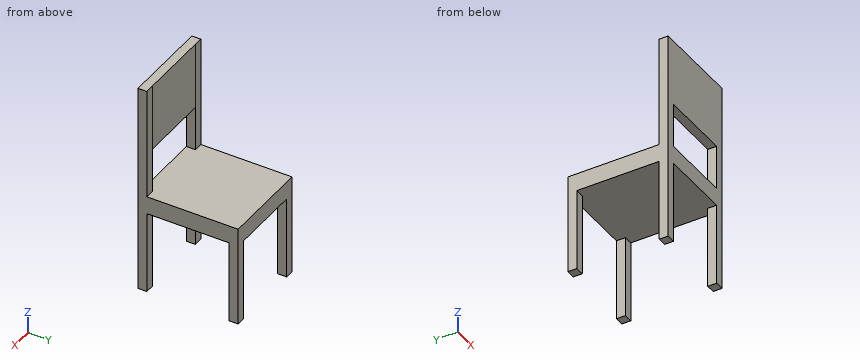
```python
from build123d import *

# Parameters (mm, degrees)
F0_W     = 400
F0_H     = 450
F1_DEPTH = 80
F2_W     = 40
F2_H     = 40
F3_DEPTH = 500
F4_DEPTH = 450
F5_W     = 360
F5_H     = 39.547034
F6_DEPTH = 300


with BuildPart() as f1:
    # F0 (on Top) → F1 (new body)
    with BuildSketch(Plane.XY):
        with Locations((200, 225)):
            Rectangle(F0_W, F0_H)
    extrude(amount=-F1_DEPTH)

    # F2 (on face) → F3 (join)
    with BuildSketch(Plane.XY):
        with Locations((20, 20)):
            Rectangle(F2_W, F2_H)
        with Locations((380, 20)):
            Rectangle(F2_W, F2_H)
    extrude(amount=F3_DEPTH)

    # F2 (on face) → F4 (join)
    with BuildSketch(Plane.XY):
        with Locations((20, 20)):
            Rectangle(F2_W, F2_H)
        with Locations((380, 20)):
            Rectangle(F2_W, F2_H)
        with Locations((380, 430)):
            Rectangle(F2_W, F2_H)
        with Locations((20, 430)):
            Rectangle(F2_W, F2_H)
    extrude(amount=-F4_DEPTH)

    # F5 (on face) → F6 (join)
    with BuildSketch(Plane.XY.offset(500)):
        with Locations((220, 19.773517)):
            Rectangle(F5_W, F5_H)
    extrude(amount=-F6_DEPTH)


solid = f1.part
```
Work out the finished part from the listing and answer in its coordinate system (mm). Coordinates: 2 decimals unless noted, no trailing zeros. Order: outer loops, then holes, each group sorted by start corner. A loop starts at its lowest first (then second) coordinate and runs counter-clockwise, first axis right, second up. Notation, with made-up numbers: (-8, 81) - (45, 81) arc R25 cw to (45, 93) - close; hole circle Ø5 at (84.5, 87). An arc over 180 degrees is marked (long way). Answer as a JSON object with one key per item and string values.
1. Find section B-B on z = -217.5. Determine the outline of the cut face in (x, y), plus the area to 3 significant figures.
Output values:
{"outline": "(0, 0) - (40, 0) - (40, 40) - (0, 40) - close; (0, 410) - (40, 410) - (40, 450) - (0, 450) - close; (360, 0) - (400, 0) - (400, 40) - (360, 40) - close; (360, 410) - (400, 410) - (400, 450) - (360, 450) - close", "area": "6,400 mm²"}
2. Find section C-C on x = 227. Determine the outline of the cut face in (y, z), plus the area to 3 significant figures.
Output values:
{"outline": "(0, -80) - (450, -80) - (450, 0) - (0, 0) - close; (0, 200) - (39.55, 200) - (39.55, 500) - (0, 500) - close", "area": "47,900 mm²"}
3. Each of these flat-tipped pins is pushed along its axis until it touches: P1, Ø5, axis at x = 145.5, y = 74, coming from the +Z side; P2, Ø20, axis at x = 25.5, z = 296, coming from the +Y side. Where does it stop, or does it pass through?
Output values:
{"P1": "stops at z = 0", "P2": "stops at y = 40"}
4. Consider line 1 (Y direction, x = 376.5, z = -149); line 2 (X direction, y = 27, z = 119); line 3 (Z direction, x = 320.5, y = 358.5). Determine where each line is inside the solid, lowest interval first.
Output values:
{"line 1": "y = 0 to 40, 410 to 450", "line 2": "x = 0 to 40, 360 to 400", "line 3": "z = -80 to 0"}
5. Find section A-A on z = 54. Determine the outline of the cut face in (x, y).
Output values:
{"outline": "(0, 0) - (40, 0) - (40, 40) - (0, 40) - close; (360, 0) - (400, 0) - (400, 40) - (360, 40) - close"}
6. Find section D-D on z = 353. Determine the outline of the cut face in (x, y).
Output values:
{"outline": "(0, 0) - (400, 0) - (400, 40) - (360, 40) - (360, 39.55) - (40, 39.55) - (40, 40) - (0, 40) - close"}
